Geometry check sheet. Reference: the model listing, model coordinates, mm. Face numbers are marked on the shaded views. A direction names the side the tool comes from. Coordinates: 2 decimals unless noted, no trailing zeros. Answer in a Markdown table with one row per item. Add a question column.
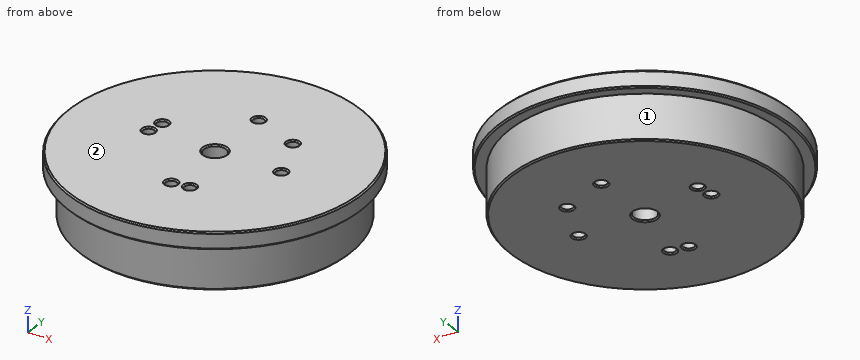
```python
from build123d import *

# Parameters (mm, degrees)
SKETCH1_R           = 76.073
BOSS_EXTRUDE1_DEPTH = 25.4
SKETCH2_R           = 82.55
BOSS_EXTRUDE2_DEPTH = 9.525
SKETCH3_R           = 3.175
CUT_EXTRUDE1_DEPTH  = 122.855490746
SKETCH5_R           = 6.35
CUT_EXTRUDE2_DEPTH  = 122.855490746
CHAMFER1_SIZE       = 0.762


with BuildPart() as part:
    # Sketch1 → Boss-Extrude1 (new body)
    with BuildSketch(Plane.XY):
        Circle(SKETCH1_R)
    extrude(amount=BOSS_EXTRUDE1_DEPTH)

    # Sketch2 → Boss-Extrude2 (add)
    with BuildSketch(Plane.XY.offset(25.4)):
        with Locations(Location((0, 0, 0), (0, 0, 180))):
            Circle(SKETCH2_R)
    extrude(amount=BOSS_EXTRUDE2_DEPTH)

    # Sketch3 → Cut-Extrude1 (cut, through all)
    with BuildSketch(Plane.XY.offset(34.925)):
        with Locations((0, 38.1)):
            Circle(SKETCH3_R)
        with Locations((26.940768363, 26.940768363)):
            Circle(SKETCH3_R)
        with Locations((38.1, 0)):
            Circle(SKETCH3_R)
        with Locations((9.861005618, -36.801773982)):
            Circle(SKETCH3_R)
        with Locations((0, -38.1)):
            Circle(SKETCH3_R)
        with Locations((-38.1, 0)):
            Circle(SKETCH3_R)
        with Locations((-36.801773982, 9.861005618)):
            Circle(SKETCH3_R)
    extrude(amount=-CUT_EXTRUDE1_DEPTH, mode=Mode.SUBTRACT)

    # Sketch5 → Cut-Extrude2 (cut, through all)
    with BuildSketch(Plane.XY.offset(34.925)):
        Circle(SKETCH5_R)
    extrude(amount=-CUT_EXTRUDE2_DEPTH, mode=Mode.SUBTRACT)

    # Chamfer1
    chamfer1_edges = [part.edges().sort_by_distance(p)[0] for p in [
        (-76.073, 0, 0),
        (-39.976773982, 9.861005618, 0),
        (-39.976773982, 9.861005618, 34.925),
        (-41.275, 0, 0),
        (-41.275, 0, 34.925),
        (-3.175, -38.1, 0),
        (-3.175, -38.1, 34.925),
        (6.686005618, -36.801773982, 0),
        (6.686005618, -36.801773982, 34.925),
        (-3.175, 38.1, 0),
        (-3.175, 38.1, 34.925),
        (34.925, 0, 0),
        (34.925, 0, 34.925),
        (23.765768363, 26.940768363, 0),
        (23.765768363, 26.940768363, 34.925),
        (-6.35, 0, 0),
        (-6.35, 0, 34.925),
        (82.55, 0, 25.4),
        (82.55, 0, 34.925),
    ]]
    chamfer(chamfer1_edges, length=CHAMFER1_SIZE)


solid = part.part
```
(1) Scan lines: line 1 along Y through (x, z) = (0, 10) (3 decimals); line 2 along Y through (x, z) = (-38, 17); line 3 along Y through (x, z) = (-38.1, 25) (3 decimals). Record each from-to range of solid material in increasing order.
(2) Access from +Z, -Z, +X, -X, +Y, -Y to the whole of each face (thin tool, end or side, straight path). Record for the marked faces 1 and 2.
(3) Go/stop test with flat-tipped pins: P1, Ø6, axis at x = 36, y = -39, coming from the -Z side; P2, Ø3, axis at y = -50.5, z = 23, coming from the +X side; P3, Ø3, axis at x = -33, z = 31, coming from the -Y side; P4, Ø2, axis at y = 22.5, z = 22.5, coming from the +X side. Record where each tip stops, or that it passes through.
(4) Cross-section at A-A (z = 30.5). Give the number of separate pieces and of enclosed holes in the cut face, plus the area to 3 significant figures.
Checks:
| question | item | result |
|---|---|---|
| 1 | line 1 | -76.073 to -41.275, -34.925 to -6.35, 6.35 to 34.925, 41.275 to 76.073 |
| 1 | line 2 | -65.9 to -3.17, 3.17 to 6.92, 12.8 to 65.9 |
| 1 | line 3 | -65.844 to -3.175, 3.175 to 6.964, 12.758 to 65.844 |
| 2 | face 1 | -Z |
| 2 | face 2 | +Z, +X, -X, +Y, -Y |
| 3 | P1 | z = 0 |
| 3 | P2 | x = 58.19 |
| 3 | P3 | y = -76.3 |
| 3 | P4 | x = 72.97 |
| 4 | separate pieces | 1 |
| 4 | enclosed holes | 8 |
| 4 | area | 21,100 mm² |
